Read the model definition and answer for the solid it produces. Units are mm, in the model's axes. A direction names the side the tool comes from. Round coordinates to 2 decimals unless told otherwise and drop trailing zeros. Loops run counter-clockwise (first coordinate to the right, second up) from the corner with the lowest first, then second, coordinate; pieces in that order, holes last. Notation, with made-up numbers: (28, 3) - (82, 3) arc R23 cw to (82, 28) - close; hole circle Ø10 at (-2.75, 2.25). An arc over 180 degrees is marked (long way). Answer as CSV lines item,"result".
```python
from build123d import *
from build123d.topology import SkipClean

# Parameters (mm, degrees)
SKETCH_2_W                 = 150
SKETCH_2_H                 = 60
EXTRUDE_1_DEPTH            = 5
SKETCH_3_W                 = 15
SKETCH_3_H                 = 20
EXTRUDE_2_DEPTH            = 150
PATTERN_LINEAR_1_COUNT     = 2
PATTERN_LINEAR_1_PITCH     = 25
PATTERN_LINEAR_1_COL_COUNT = 2
PATTERN_LINEAR_1_COL_PITCH = 25
SKETCH_22_R                = 4
CUT_EXTRUDE_3_DEPTH        = 5
MIRROR_19_COPY_1_SKETCH_R  = 4
MIRROR_19_COPY_1_DEPTH     = 5


with BuildPart() as part:
    # 草图2 → 凸台-拉伸1 (new body)
    with BuildSketch(Plane(origin=(0, 0, 0), x_dir=(1, 0, 0), z_dir=(0, 1, 0))):
        with Locations((-40.476378725, 10.538808084)):
            Rectangle(SKETCH_2_W, SKETCH_2_H)
    extrude(amount=EXTRUDE_1_DEPTH)

    # 草图3 → 凸台-拉伸2 (add)
    with BuildSketch(Plane(origin=(0, 0, 0), x_dir=(1, 0, 0), z_dir=(0, 1, 0))):
        with Locations((-97.302512432, 10.572361891)):
            Rectangle(SKETCH_3_W, SKETCH_3_H)
    extrude_2 = extrude(amount=EXTRUDE_2_DEPTH)

    # 草图19 → 切除-旋转29 (revolve, cut)
    with BuildSketch(Plane.XY.offset(-10.538808084)):
        with BuildLine():
            Line((-89.802512432, 90.57618696), (-89.802512432, 75.771839239))
            ThreePointArc((-89.802512432, 75.771839239), (-97.204686292, 83.1740131), (-89.802512432, 90.57618696))
        make_face()
    cut_revolve_29 = revolve(axis=Axis((-89.802512432, 90.57618696, -10.538808084), (0, -1, 0)), mode=Mode.SUBTRACT)

    # 阵列(线性)1: 切除-旋转29 ×2
    with Locations(*[(0, i * PATTERN_LINEAR_1_PITCH, 0) for i in range(1, PATTERN_LINEAR_1_COUNT)]):
        add(cut_revolve_29, mode=Mode.SUBTRACT)

    # 阵列(线性)1 col: 切除-旋转29 ×2
    with Locations(*[(0, -i * PATTERN_LINEAR_1_COL_PITCH, 0) for i in range(1, PATTERN_LINEAR_1_COL_COUNT)]):
        add(cut_revolve_29, mode=Mode.SUBTRACT)

    # 草图22 → 切除-拉伸3 (cut)
    with BuildSketch(Plane(origin=(0, 0, 0), x_dir=(1, 0, 0), z_dir=(0, 1, 0))):
        with Locations(Location((-109.062885819, 34.038808084, 0), (0, 0, 270))):
            Circle(SKETCH_22_R)
    cut_extrude_3 = extrude(amount=CUT_EXTRUDE_3_DEPTH, mode=Mode.SUBTRACT)

    # 镜向18: 切除-拉伸3 across plane
    add(cut_extrude_3.mirror(Plane.XY.offset(-10.538808084)), mode=Mode.SUBTRACT)

    # 镜向19: 切除-拉伸3 across plane
    add(cut_extrude_3.mirror(Plane(origin=(-40.476378725, 0, 0), x_dir=(0, 0, 1), z_dir=(1, 0, 0))), mode=Mode.SUBTRACT)

    # 镜向19 copy 1 sketch → 镜向19 copy 1 (cut)
    with BuildSketch(Plane(origin=(-80.95275745, 0, -21.077616169), x_dir=(-1, 0, 0), z_dir=(0, 1, 0))):
        with Locations(Location((-109.062885819, 34.038808084, 0), (0, 0, 270))):
            Circle(MIRROR_19_COPY_1_SKETCH_R)
    extrude(amount=MIRROR_19_COPY_1_DEPTH, mode=Mode.SUBTRACT)

    # 镜向20: 凸台-拉伸2 across plane
    add(extrude_2.mirror(Plane(origin=(-40.476378725, 0, 0), x_dir=(0, 0, 1), z_dir=(1, 0, 0))))

    # 镜向21: 切除-旋转29 across plane
    with SkipClean():  # the faces are left unmerged after this step: merging them gives an invalid solid
        add(cut_revolve_29.mirror(Plane(origin=(-40.476378725, 0, 0), x_dir=(0, 0, 1), z_dir=(1, 0, 0))), mode=Mode.SUBTRACT)

    # 镜向22 copy 1 sketch → 镜向22 copy 1 (revolve, cut)
    with SkipClean():  # the faces are left unmerged after this step: merging them gives an invalid solid
        with BuildSketch(Plane(origin=(-80.95275745, 25, -10.538808084), x_dir=(-1, 0, 0), z_dir=(0, 0, 1))):
            with BuildLine():
                Line((-89.802512432, -90.57618696), (-89.802512432, -75.771839239))
                ThreePointArc((-89.802512432, -75.771839239), (-97.204686292, -83.1740131), (-89.802512432, -90.57618696))
            make_face()
        revolve(axis=Axis((8.849754981, 115.57618696, -10.538808084), (0, 1, 0)), mode=Mode.SUBTRACT)

    # 镜向22 copy 2 sketch → 镜向22 copy 2 (revolve, cut)
    with SkipClean():  # the faces are left unmerged after this step: merging them gives an invalid solid
        with BuildSketch(Plane(origin=(-80.95275745, -25, -10.538808084), x_dir=(-1, 0, 0), z_dir=(0, 0, 1))):
            with BuildLine():
                Line((-89.802512432, -90.57618696), (-89.802512432, -75.771839239))
                ThreePointArc((-89.802512432, -75.771839239), (-97.204686292, -83.1740131), (-89.802512432, -90.57618696))
            make_face()
        revolve(axis=Axis((8.849754981, 65.57618696, -10.538808084), (0, 1, 0)), mode=Mode.SUBTRACT)

    # 镜向22 copy 3 sketch → 镜向22 copy 3 (revolve, cut)
    with SkipClean():  # the faces are left unmerged after this step: merging them gives an invalid solid
        with BuildSketch(Plane(origin=(-80.95275745, 0, -10.538808084), x_dir=(-1, 0, 0), z_dir=(0, 0, 1))):
            with BuildLine():
                Line((-89.802512432, -90.57618696), (-89.802512432, -75.771839239))
                ThreePointArc((-89.802512432, -75.771839239), (-97.204686292, -83.1740131), (-89.802512432, -90.57618696))
            make_face()
        revolve(axis=Axis((8.849754981, 90.57618696, -10.538808084), (0, 1, 0)), mode=Mode.SUBTRACT)


solid = part.part
```
1) A tool of negligible diameter and unlimited length cuts with its end or side. For faces 1 (the face through (16, 76, -0.572)), 2 (the face through (8.85, 76, -15)), 3 (the face through (16, 76, -20.572)), from which of +Z, -Z, +X, -X, +Y, -Y can it reach the whole face along a straight path? Write none if from no direction.
Entries:
face 1,"+Z, +X, -X, +Y"
face 2,"+Z, -Z, +Y"
face 3,"-Z, +X, -X, +Y"
2) Each of these flat-tipped pins is pushed along its axis until it touches: P1, Ø10.5, axis at x = -109.06, z = -34.04, coming from the +Y side; P2, Ø12, axis at x = -96, y = 81.5, coming from the +Z side; P3, Ø16, axis at y = 64, z = -11.5, coming from the -X side; P4, Ø5, axis at x = -109.06, z = 12.96, coming from the +Y side. Where does it stop, or does it pass through?
Entries:
P1,"stops at y = 5"
P2,"stops at z = -0.57"
P3,"stops at x = -104.8"
P4,"passes through"
3) A cutting plane is placed at D-D, the plane z = -27. Determine the outline of the cut face in (x, y), plus the area to 3 significant figures.
Entries:
outline,"(-115.48, 0) - (34.52, 0) - (34.52, 5) - (-115.48, 5) - close"
area,"750 mm^2"
4) A cutting plane is placed at C-C, the plane x = -71. Determine the outline of the cut face in (y, z), plus the area to 3 significant figures.
Entries:
outline,"(0, -40.54) - (5, -40.54) - (5, 19.46) - (0, 19.46) - close"
area,"300 mm^2"
5) Find the intervals of material crossed by line 1 (X direction, y = 56.5, z = -18); line 2 (Y direction, x = -24, z = 17); line 3 (Z direction, x = 17.5, y = 86), in increasing order.
Entries:
line 1,"x = -104.8 to -89.8, 8.85 to 23.85"
line 2,"y = 0 to 5"
line 3,"z = -20.57 to -0.57"
6) A cutting plane is placed at B-B, the plane z = -36. Determine the outline of the cut face in (x, y).
Entries:
outline,"(-115.48, 0) - (-112.55, 0) - (-112.55, 5) - (-115.48, 5) - close; (-105.58, 0) - (24.62, 0) - (24.62, 5) - (-105.58, 5) - close; (31.6, 0) - (34.52, 0) - (34.52, 5) - (31.6, 5) - close"
7) The mould has two halves that part along X. Classify faces 4 (the face through (26.909, 2.465, -30.224)), 5 (the face through (-115.476, 2, -10)), 6 (the face through (-39, 0, -11)), 7 (the face through (-112.612, 2.465, 11.115)): pulls with the +X half, pulls with the -X half, needs draft (parallel to the pull), parting line crosses it, or undercut.
Entries:
face 4,"undercut"
face 5,"pulls with the -X half"
face 6,"needs draft"
face 7,"undercut"
8) A cutting plane is placed at A-A, the plane y = 69. Determine the outline of the cut face in (x, z).
Entries:
outline,"(-104.8, -20.57) - (-89.8, -20.57) - (-89.8, -0.57) - (-104.8, -0.57) - close; (8.85, -20.57) - (23.85, -20.57) - (23.85, -0.57) - (8.85, -0.57) - close"
